Autodesk Fusion 360 part; units mm, degrees
sketch "Sketch1" plane through (0, 0, 0) normal (1, 0, 0) x (0, 0, -1)
  line L0 (0, 40) -> (-2, 40)
  line L1 (-2, 40) -> (-2, 0)
  line L2 (-2, 0) -> (0, 0)
  line L3 (0, 0) -> (0, 40)
  line L4 (0, 0) -> (-40, 0)
  line L5 (-40, 0) -> (-40, 2)
  line L6 (-40, 2) -> (0, 2)
  line L7 (0, 2) -> (0, 0)
  dimension "d1" = 2
  dimension "d2" = 40
extrude "Extrude1" add sketch "Sketch1" along normal blind 40
sketch "Sketch2" plane through (0, 0, 0) normal (0, 0, -1) x (-1, 0, 0)
  circle A0 centre (-20, 13) radius 2
  circle A1 centre (-10.4737, 29.5) radius 2
  circle A2 centre (-29.5263, 29.5) radius 2
  point P0 (-20, 24)
  dimension "d5" = 4
  dimension "d8" = 360
extrude "Extrude2" cut sketch "Sketch2" against normal blind 2
ref_plane "WorkPlane1" through (0, 2, 2) normal (0, -0.7071, 0.7071) x (1, 0, 0)
mirror "Mirror1" about plane through (0, 2, 2) normal (0, -0.7071, 0.7071) of "Extrude2"
Verification items for the finished model (mm, model axes). A direction names the side the tool comes from. Round coordinates to 2 decimals unless told otherwise and drop trailing zeros. Write each loop counter-clockwise with the first axis right and the second up, starting at its lowest first coordinate (ties: lowest second). Pieces come first, ordered by that corner, then holes. Notation, with made-up numbers: (-10, 45) -> (41, 45) arc R18 cw to (41, 73) -> close; hole circle Ø8 at (68.25, 74.25). An arc over 180 degrees is marked (long way). Write each question's results on one line, items separated by ' | '. Start each with the question number.
1. Depth check by flat-ended pin: P1, Ø3, axis at x = 29.53, z = 29.5, coming from the -Y side; P2, Ø5, axis at x = 10.47, z = 29.5, coming from the +Y side; P3, Ø2, axis at x = 19, y = 9, coming from the +Z side. Enter the tip coordinate at first touch or a pass-through.
2. Material ranges on probe 1 along Z at (x, y) = (24, 31), recorded low to high. Write a range as from..to.
3. Cross-section at D-D (x = 29). Enter the section's corners in (y, z).
4. Cross-section at A-A (y = 29.5). Enter the section's corners in (x, z), then the cut area to 3 significant figures.
5. Draft check along Y on faces 1 (the flat face through (20, 0, 20)), 2 (the cylindrical face through (21.474, 14.352, 0.986)), 3 (the cylindrical face through (28.603, 27.726, 0.986)), 4 (the cylindrical face through (21.474, 0.986, 11.648)). Enter one of: +Y half, -Y half, draft (parallel to the pull), parting line (faces both ways), or undercut.
6. Set-up check for faces 5 (the flat face through (20, 21, 2)), 6 (the cylindrical face through (28.603, 0.986, 31.274)): record each of +Z, -Z, +X, -X, +Y, -Y from which the full face is reachable in a straight line by a thin tool's end or side.
7. Cross-section at C-C (y = 13). Enter the section's corners in (x, z), then the cut area to 3 significant figures.
Solutions:
1) P1: passes through | P2: stops at y = 2 | P3: stops at z = 2
2) probe 1: z = 0..2
3) outline: (0, 0) -> (27.57, 0) -> (27.57, 2) -> (2, 2) -> (2, 27.57) -> (0, 27.57) -> close; (0, 31.43) -> (2, 31.43) -> (2, 40) -> (0, 40) -> close; (31.43, 0) -> (40, 0) -> (40, 2) -> (31.43, 2) -> close
4) outline: (0, 0) -> (8.47, 0) -> (8.47, 2) -> (0, 2) -> close; (12.47, 0) -> (27.53, 0) -> (27.53, 2) -> (12.47, 2) -> close; (31.53, 0) -> (40, 0) -> (40, 2) -> (31.53, 2) -> close | area: 64.0 mm2
5) face 1: -Y half | face 2: undercut | face 3: undercut | face 4: draft
6) face 5: +Z, +X, -X, +Y | face 6: +Y, -Y
7) outline: (0, 0) -> (18, 0) -> (18, 2) -> (0, 2) -> close; (22, 0) -> (40, 0) -> (40, 2) -> (22, 2) -> close | area: 72.0 mm2
